Verification items for the finished model (mm, model axes). A direction names the side the tool comes from. Coordinates: 2 decimals unless noted, no trailing zeros. Order: outer loops, then holes, each group sorted by start corner. A loop starts at its lowest first (then second) coordinate and runs counter-clockwise, first axis right, second up. Notation, with made-up numbers: (-25.75, 36.5) -> (26.25, 36.5) arc R19 cw to (26.25, 41.5) -> close; hole circle Ø4 at (-34, -23). An arc over 180 degrees is marked (long way). Use CSV: the item, a comma, the result in double quotes. Start each with the question number.
1) Release check for a two-part mould opening along Y. For faces 1 (the flat face through (-3.295, 54.12, 0.042)), 2 (the flat face through (-3.205, 21.85, 0.042)), 3 (the flat face through (30, 47, 0)) record: released by +Y, released by -Y, zero draft, split by the parting line, or undercut.
2) Go/stop test with flat-tipped pins: pin 1 (1.6 mm diameter, centred on y = 66.5, z = 0, fed in from -X); pin 2 (1 mm diameter, centred on x = -1.5, z = -1, fed in from +Y). Record where each tip stops, or that it passes through.
3) Sectioned sample at C-C on y = 85.5. Record the boundary of the cut face in (x, z).
4) Sectioned sample at D-D on x = 22.5. Record the boundary of the cut face in (y, z).
5) Sectioned sample at B-B on x = -2. Give the number of separate pieces and of enclosed holes in the cut face, then the cut area to 3 significant figures.
6) Tool access check on faces 4 (the flat face through (13, 20, 0)), 5 (the flat face through (-3.205, 69.378, 0.042)). Record the directions out of +Z, -Z, +X, -X, +Y, -Y that give a thin tool (end or side, any length) a straight path to the whole face; none if there is none.
7) Scan lines: line 1 along X through (y, z) = (67, 1.5); line 2 along X through (y, z) = (24, 2.75); line 3 along Y through (x, z) = (1, 2.5). Record each from-to range of solid material in increasing order.
from build123d import *

# Parameters (mm, degrees)
SALIENTE_EXTRUIR1_DEPTH = 3
SALIENTE_EXTRUIR3_DEPTH = 6
REDONDEO1_R             = 5


with BuildPart() as part:
    # Croquis1 → Saliente-Extruir1 (new, symmetric)
    with BuildSketch(Plane.XY):
        Polygon((0, 20), (0, 100), (30, 70), (30, 20), align=None)
    extrude(amount=SALIENTE_EXTRUIR1_DEPTH, both=True)

    # Croquis4 → Saliente-Extruir3 (add, through all)
    with BuildSketch(Plane.XY.offset(3)):
        Polygon((0, 20), (-6.5, 23.75277675), (0, 27.505553499), align=None)
        Polygon((0, 37.011106999), (0, 29.505553499), (-6.5, 33.258330249), align=None)
        Polygon((0, 46.516660498), (0, 39.011106999), (-6.5, 42.763883749), align=None)
        Polygon((0, 56.022213998), (0, 48.516660498), (-6.5, 52.269437248), align=None)
        Polygon((0, 65.527767497), (0, 58.022213998), (-6.5, 61.774990748), align=None)
        Polygon((0, 75.033320997), (0, 67.527767497), (-6.5, 71.280544247), align=None)
        Polygon((0, 84.538874496), (0, 77.033320997), (-6.5, 80.786097747), align=None)
        Polygon((0, 94.044427996), (0, 86.538874496), (-6.5, 90.291651246), align=None)
    extrude(amount=-SALIENTE_EXTRUIR3_DEPTH)

    # Redondeo1
    # the kernel refuses this fillet: 5 mm, written as the material it takes off along each edge
    with BuildSketch(Plane(origin=(0, 100, 25.871542056), x_dir=(0, -1, 0), z_dir=(0, 0, -1))) as redondeo1_piece_1:
        with BuildLine():
            CenterArc((10.0045829, -2.933515088), REDONDEO1_R, 144.076608278, 80.923391722)
            Line((6.469048994, -6.469048994), (6.398338316, -6.539759672))
            Line((6.398338316, -6.539759672), (-0.070710678, -0.070710678))
            Line((-0.070710678, -0.070710678), (0, 0.1))
            ThreePointArc((0, 0.1), (2.977786002, 0.1), (5.874591786, 0.058670302))
            Line((5.874591786, 0.058670302), (5.955572004, 0))
        make_face()
    extrude(amount=51.743084112, mode=Mode.SUBTRACT)
    with BuildSketch(Plane(origin=(30, 20, -15.5), x_dir=(0, 1, 0), z_dir=(0, 0, 1))) as redondeo1_piece_2:
        with BuildLine():
            CenterArc((REDONDEO1_R, REDONDEO1_R), REDONDEO1_R, 180, 90)
            Line((0, REDONDEO1_R), (-REDONDEO1_R * 0.02, REDONDEO1_R))
            Line((-REDONDEO1_R * 0.02, REDONDEO1_R), (-REDONDEO1_R * 0.02, -REDONDEO1_R * 0.02))
            Line((-REDONDEO1_R * 0.02, -REDONDEO1_R * 0.02), (REDONDEO1_R, -REDONDEO1_R * 0.02))
            Line((REDONDEO1_R, -REDONDEO1_R * 0.02), (REDONDEO1_R, 0))
        make_face()
    extrude(amount=31, mode=Mode.SUBTRACT)
    with BuildSketch(Plane(origin=(30, 70, 8.17766953), x_dir=(-0.7071067811865449, 0.70710678118655, 0), z_dir=(0, 0, -1))) as redondeo1_piece_3:
        with BuildLine():
            CenterArc((REDONDEO1_R * 0.414213562373, -REDONDEO1_R), REDONDEO1_R, 90, 45)
            Line((-REDONDEO1_R * 0.292893218813, -REDONDEO1_R * 0.292893218813), (-REDONDEO1_R * 0.307035354437, -REDONDEO1_R * 0.27875108319))
            Line((-REDONDEO1_R * 0.307035354437, -REDONDEO1_R * 0.27875108319), (-REDONDEO1_R * 0.00828427124746, REDONDEO1_R * 0.02))
            Line((-REDONDEO1_R * 0.00828427124746, REDONDEO1_R * 0.02), (REDONDEO1_R * 0.414213562373, REDONDEO1_R * 0.02))
            Line((REDONDEO1_R * 0.414213562373, REDONDEO1_R * 0.02), (REDONDEO1_R * 0.414213562373, 0))
        make_face()
    extrude(amount=16.355339059, mode=Mode.SUBTRACT)


solid = part.part
Answers follow:
1,face 1,"undercut"
1,face 2,"released by -Y"
1,face 3,"zero draft"
2,pin 1,"stops at x = 0"
2,pin 2,"stops at y = 93.47"
3,outline,"(0, -3) -> (14.5, -3) -> (14.5, 3) -> (0, 3) -> close"
4,outline,"(20, -3) -> (77.5, -3) -> (77.5, 3) -> (20, 3) -> close"
5,separate pieces,"8"
5,enclosed holes,"0"
5,area,"249 mm²"
6,face 4,"+Z, -Z, +X, -X, -Y"
6,face 5,"+Z, -Z, -X"
7,line 1,"x = 0 to 30"
7,line 2,"x = -6.07 to 29.9"
7,line 3,"y = 20 to 94.61"
